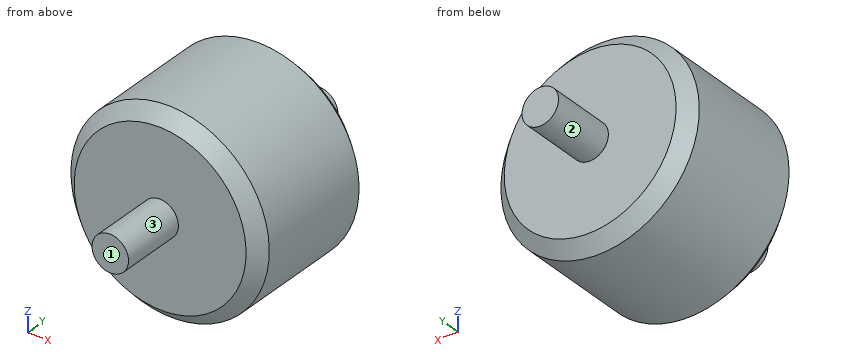
from build123d import *

# Parameters (mm, degrees)
SKETCH1_W   = 9.525
SKETCH1_H   = 11.43
SKETCH1_W_2 = 1.7526
SKETCH1_H_2 = 6.35


with BuildPart() as part:
    # Sketch1 → Revolve1 (revolve)
    with BuildSketch(Plane(origin=(0, 0, 0), x_dir=(0, 0, -1), z_dir=(1, 0, 0))):
        with Locations((4.7625, -5.715)):
            Rectangle(SKETCH1_W, SKETCH1_H)
        Polygon((1.27, 1.27), (0, 0), (9.525, 0), (9.525, 1.27), (7.7724, 1.27), align=None)
        with Locations((8.6487, 4.445)):
            Rectangle(SKETCH1_W_2, SKETCH1_H_2)
        Polygon((9.525, -11.43), (0, -11.43), (1.27, -12.7), (7.7724, -12.7), (9.525, -12.7), align=None)
        with Locations((8.6487, -15.875)):
            Rectangle(SKETCH1_W_2, SKETCH1_H_2)
    revolve(axis=Axis((0, 7.62, -9.525), (0, -1, 0)))


solid = part.part
Work out the finished part from the listing and answer in its coordinate system (mm). Face numbers are marked on the shaded views. A direction names the side the tool comes from. Give positions to 0.01 mm unless a question says otherwise; leave off trailing zeros. Write each loop counter-clockwise with the first axis right and the second up, starting at its lowest first coordinate (ties: lowest second). Pieces come first, ordered by that corner, then holes. Notation, with made-up numbers: (32, 17.25) - (78, 17.25) arc R28 cw to (78, 41.25) - close; hole circle Ø5 at (69, 43). An arc over 180 degrees is marked (long way). One line per item, written item: value. Start each with the question number.
1. Given pin 1 (6 mm diameter, centred on x = 2.5, y = -15, fed in from -Z); pin 2 (1.5 mm diameter, centred on y = -8, z = -7.5, fed in from -X); pin 3 (1 mm diameter, centred on x = 7, z = -16, fed in from +Y), each flat-ended and moving along its own axis, determine where each tip first touches the part or whether it passes through.
2. Consider probe 1 along Y at (x, z) = (0.25, -4.75); probe 2 along Z at (x, y) = (-8.5, -10.25); probe 3 along X at (y, z) = (-7.25, -3). Determine where each line is inside the solid, lowest interval first.
3. Find section C-C (y = -14.5). Write down the section's boundary in (x, z) (3 decimals), then the cut area to 3 significant figures.
4. For the marked faces 1, 2 and 3, determine the directions among +Z, -Z, +X, -X, +Y, -Y from which every point of the face is accessible in a straight line to the end or side of a thin tool.
5. Find section B-B (y = -6.5). Write down the section's boundary in (x, z) (3 decimals), then the cut area to 3 significant figures.
6. Find section A-A (x = 0). Write down the section's boundary in (y, z).
Geometry results:
1. pin 1: z = -18.21
1. pin 2: x = -9.44
1. pin 3: y = 0.49
2. probe 1: -12.7 to 1.27
2. probe 2: -13.82 to -5.23
2. probe 3: -6.94 to 6.94
3. outline: circle Ø3.505 at (0, -9.525)
3. area: 9.65 mm2
4. face 1: +Z, -Z, +X, -X, -Y
4. face 2: +Y
4. face 3: -Y
5. outline: circle Ø19.05 at (0, -9.525)
5. area: 285 mm2
6. outline: (-19.05, -11.28) - (-12.7, -11.28) - (-12.7, -17.78) - (-11.43, -19.05) - (0, -19.05) - (1.27, -17.78) - (1.27, -11.28) - (7.62, -11.28) - (7.62, -7.77) - (1.27, -7.77) - (1.27, -1.27) - (0, 0) - (-11.43, 0) - (-12.7, -1.27) - (-12.7, -7.77) - (-19.05, -7.77) - close
